```python
from build123d import *

# Parameters (mm, degrees)
SKETCH1_W           = 40
SKETCH1_H           = 20
BOSS_EXTRUDE1_DEPTH = 39
BOSS_EXTRUDE2_DEPTH = 2.5
FILLET1_R           = 2.5
SKETCH3_R           = 5
BOSS_EXTRUDE3_DEPTH = 2.5
SKETCH4_R           = 2.5
BOSS_EXTRUDE4_DEPTH = 4
FILLET2_R           = 2.5
FILLET3_R           = 2.5


with BuildPart() as part:
    # Sketch1 → Boss-Extrude1 (new body)
    with BuildSketch(Plane(origin=(0, 0, 0), x_dir=(1, 0, 0), z_dir=(0, 1, 0))):
        with Locations((20, 10)):
            Rectangle(SKETCH1_W, SKETCH1_H)
    extrude(amount=BOSS_EXTRUDE1_DEPTH)

    # Sketch2 → Boss-Extrude2 (add)
    with BuildSketch(Plane(origin=(0, 28.9, 0), x_dir=(-1, 0, 0), z_dir=(0, -1, 0))):
        with BuildLine():
            ThreePointArc((-44.8, 12.5), (-46.382129215, 13.064317395), (-47.25, 14.502506281))
            Line((-47.25, 14.502506281), (-47.25, 5.497493719))
            ThreePointArc((-47.25, 5.497493719), (-46.382129215, 6.935682605), (-44.8, 7.5))
            Line((-44.8, 7.5), (-44.8, 12.5))
        make_face()
        with BuildLine():
            Line((7.25, 20), (-47.25, 20))
            Line((-47.25, 20), (-47.25, 15.497493719))
            ThreePointArc((-47.25, 15.497493719), (-44.55, 17.487468593), (-42.3, 15))
            ThreePointArc((-42.3, 15), (-43.032233047, 13.232233047), (-44.8, 12.5))
            Line((-44.8, 12.5), (-44.8, 7.5))
            ThreePointArc((-44.8, 7.5), (-43.032233047, 6.767766953), (-42.3, 5))
            ThreePointArc((-42.3, 5), (-44.55, 2.512531407), (-47.25, 4.502506281))
            Line((-47.25, 4.502506281), (-47.25, 0))
            Line((-47.25, 0), (7.25, 0))
            Line((7.25, 0), (7.25, 4.502506281))
            ThreePointArc((7.25, 4.502506281), (2.3, 5), (7.25, 5.497493719))
            Line((7.25, 5.497493719), (7.25, 14.502506281))
            ThreePointArc((7.25, 14.502506281), (2.3, 15), (7.25, 15.497493719))
            Line((7.25, 15.497493719), (7.25, 20))
        make_face()
    extrude(amount=-BOSS_EXTRUDE2_DEPTH)

    # Fillet1
    fillet1_edges = [part.edges().sort_by_distance(p)[0] for p in [
        (47.25, 30.15, -20),
        (-7.25, 30.15, 0),
        (-7.25, 30.15, -20),
        (47.25, 30.15, 0),
    ]]
    fillet(fillet1_edges, radius=FILLET1_R)

    # Sketch3 → Boss-Extrude3 (add)
    with BuildSketch(Plane(origin=(0, 39, 0), x_dir=(1, 0, 0), z_dir=(0, 1, 0))):
        with Locations(Location((29.9, 10, 0), (0, 0, 90))):
            Circle(SKETCH3_R)
    extrude(amount=BOSS_EXTRUDE3_DEPTH)

    # Sketch4 → Boss-Extrude4 (add)
    with BuildSketch(Plane(origin=(0, 41.5, 0), x_dir=(1, 0, 0), z_dir=(0, 1, 0))):
        with Locations(Location((29.9, 10, 0), (0, 0, 270))):
            Circle(SKETCH4_R)
    extrude(amount=BOSS_EXTRUDE4_DEPTH)

    # Fillet2
    fillet2_edges = [part.edges().sort_by_distance(p)[0] for p in [
        (0, 14.45, -20),
        (40, 14.45, -20),
        (40, 14.45, 0),
        (20, 39, -20),
        (0, 14.45, 0),
        (0, 35.2, -20),
        (40, 35.2, -20),
        (40, 35.2, 0),
        (0, 35.2, 0),
        (20, 39, 0),
    ]]
    fillet(fillet2_edges, radius=FILLET2_R)

    # Fillet3
    # the kernel refuses this fillet: 2.5 mm, written as the material it takes off along each edge
    with BuildSketch(Plane(origin=(2.5, 36.5, -2.5), x_dir=(0, 1, 0), z_dir=(-1, 0, 0))) as fillet3_piece_1_section:
        Polygon((0, 0), (FILLET3_R, 0), (FILLET3_R, -FILLET3_R), (0, -FILLET3_R), align=None)
    fillet3_piece_1 = extrude(amount=FILLET3_R, mode=Mode.PRIVATE)
    fillet3_piece_1 = fillet3_piece_1 - Plane(origin=(2.5, 36.5, -2.5), x_dir=(0, -0.7071067811865475, -0.7071067811865475), z_dir=(-1, 0, 0)) * Sphere(FILLET3_R, mode=Mode.PRIVATE)
    add(fillet3_piece_1, mode=Mode.SUBTRACT)
    with BuildSketch(Plane(origin=(37.5, 36.5, -2.5), x_dir=(1, 0, 0), z_dir=(0, 1, 0))) as fillet3_piece_2_section:
        Polygon((0, 0), (FILLET3_R, 0), (FILLET3_R, -FILLET3_R), (0, -FILLET3_R), align=None)
    fillet3_piece_2 = extrude(amount=FILLET3_R, mode=Mode.PRIVATE)
    fillet3_piece_2 = fillet3_piece_2 - Plane(origin=(37.5, 36.5, -2.5), x_dir=(-0.7071067811865475, 0, -0.7071067811865475), z_dir=(0, 1, 0)) * Sphere(FILLET3_R, mode=Mode.PRIVATE)
    add(fillet3_piece_2, mode=Mode.SUBTRACT)
    with BuildSketch(Plane(origin=(37.5, 36.5, -17.5), x_dir=(1, 0, 0), z_dir=(0, 1, 0))) as fillet3_piece_3_section:
        Polygon((0, 0), (FILLET3_R, 0), (FILLET3_R, FILLET3_R), (0, FILLET3_R), align=None)
    fillet3_piece_3 = extrude(amount=FILLET3_R, mode=Mode.PRIVATE)
    fillet3_piece_3 = fillet3_piece_3 - Plane(origin=(37.5, 36.5, -17.5), x_dir=(-0.7071067811865475, 0, 0.7071067811865475), z_dir=(0, 1, 0)) * Sphere(FILLET3_R, mode=Mode.PRIVATE)
    add(fillet3_piece_3, mode=Mode.SUBTRACT)
    with BuildSketch(Plane(origin=(2.5, 36.5, -17.5), x_dir=(0, 1, 0), z_dir=(-1, 0, 0))) as fillet3_piece_4_section:
        Polygon((0, 0), (FILLET3_R, 0), (FILLET3_R, FILLET3_R), (0, FILLET3_R), align=None)
    fillet3_piece_4 = extrude(amount=FILLET3_R, mode=Mode.PRIVATE)
    fillet3_piece_4 = fillet3_piece_4 - Plane(origin=(2.5, 36.5, -17.5), x_dir=(0, -0.7071067811865475, 0.7071067811865475), z_dir=(-1, 0, 0)) * Sphere(FILLET3_R, mode=Mode.PRIVATE)
    add(fillet3_piece_4, mode=Mode.SUBTRACT)
    with BuildSketch(Plane(origin=(0, 39, -17.5), x_dir=(0, -1, 0), z_dir=(0, 0, 1))) as fillet3_piece_5:
        with BuildLine():
            CenterArc((FILLET3_R, FILLET3_R), FILLET3_R, 180, 90)
            Line((0, FILLET3_R), (0, 0))
            Line((0, 0), (FILLET3_R, 0))
        make_face()
    extrude(amount=15, mode=Mode.SUBTRACT)
    with BuildSketch(Plane(origin=(40, 39, -2.5), x_dir=(-1, 0, 0), z_dir=(0, 0, -1))) as fillet3_piece_6:
        with BuildLine():
            CenterArc((FILLET3_R, -FILLET3_R), FILLET3_R, 90, 90)
            Line((0, -FILLET3_R), (0, 0))
            Line((0, 0), (FILLET3_R, 0))
        make_face()
    extrude(amount=15, mode=Mode.SUBTRACT)


solid = part.part
```
Can you work these out from the model? Positions are in its coordinate system, mm. A direction names the side the tool comes from. Give positions to 0.01 mm unless a question says otherwise; leave off trailing zeros. Loops run counter-clockwise (first coordinate to the right, second up) from the corner with the lowest first, then second, coordinate; pieces in that order, holes last. Notation, with made-up numbers: M 87,12.25 L 134,12.25 A8 cw 134,16.25 Z; hole C 15.5,20.5 d1. An arc over 180 degrees is marked long. Use one line per item in the form item = value. Start each with the question number.
(1) I want a section at C-C, the plane x = 29.9. Write out the boundary of the cut face in (y, z), and give its area (3 significant figures).
(2) On a 3-axis mill with a long thin cutter (end or side, diameter ignored), from which of +Z, -Z, +X, -X, +Y, -Y can I reach the whole of each face in a straight line? I mean faces 1 (the cylindrical face through (32.38, 43.47, -10.33)), 2 (the cylindrical face through (0.752, 14.652, -0.713)), 3 (the cylindrical face through (39.248, 33.986, -0.713)). Say none if no direction works.
(3) I'm going to push flat-ended pins straight in: P1, Ø4.5, axis at y = 10, z = -12.5, coming from the +X side; P2, Ø12, axis at x = 14, z = -6.5, coming from the +Y side; P3, Ø1, axis at x = -1.5, z = -11, coming from the -Y side; P4, Ø4, axis at x = -4.8, z = -15, coming from the -Y side. Where does each tip first touch, or does it pass through?
(4) Please list where these lines run through material, in increasing order: line 1 (Z direction, x = -4.8, y = 30); line 2 (Z direction, x = -4, y = 29); line 3 (X direction, y = 30.6, z = -15).
(5) I want a section at D-D, the plane z = -10. Write out the boundary of the cut face in (x, y).
(6) I want a section at B-B, the plane z = -6.25. Write out the boundary of the cut face in (x, y), and give its area (3 significant figures).
(7) I want a section at A-A, the plane y = 30.5. Write out the boundary of the cut face in (x, z).
(8) Thinking about a two-plate mould opening in Y: for faces 4 (the cylindrical face through (20.245, 38.248, -0.713)), 5 (the flat face through (20, 18, -20)), which applies, released by +Y, released by -Y, zero draft, split by the parting line, or undercut?
Worked out:
q1.outline = M 0,-20 L 36.5,-20 A2.5 ccw 39,-17.5 L 39,-15 L 41.5,-15 L 41.5,-12.5 L 45.5,-12.5 L 45.5,-7.5 L 41.5,-7.5 L 41.5,-5 L 39,-5 L 39,-2.5 A2.5 ccw 36.5,0 L 0,0 Z
q1.area = 822 mm²
q2.face_1 = +Y
q2.face_2 = +Z, -X, -Y
q2.face_3 = +Z, +X, +Y
q3.P1 = 40
q3.P2 = 39
q3.P3 = 28.9
q3.P4 = through
q4.line_1 = -20 to -17.5, -12.5 to -7.5, -2.5 to 0
q4.line_2 = -20 to -17.37, -12.63 to -7.37, -2.63 to 0
q4.line_3 = -2.3 to 42.3
q5.outline = M -7.25,28.9 L 0,28.9 L 0,0 L 40,0 L 40,28.9 L 47.25,28.9 L 47.25,31.4 L 40,31.4 L 40,36.5 A2.5 ccw 37.5,39 L 34.9,39 L 34.9,41.5 L 32.4,41.5 L 32.4,45.5 L 27.4,45.5 L 27.4,41.5 L 24.9,41.5 L 24.9,39 L 2.5,39 A2.5 ccw 0,36.5 L 0,31.4 L -7.25,31.4 Z
q6.outline = M -7.25,28.9 L -6.97,28.9 L -6.97,31.4 L -7.25,31.4 Z; M -2.63,28.9 L 0,28.9 L 0,0 L 40,0 L 40,28.9 L 42.63,28.9 L 42.63,31.4 L 40,31.4 L 40,36.5 A2.5 ccw 37.5,39 L 33.21,39 L 33.21,41.5 L 26.59,41.5 L 26.59,39 L 2.5,39 A2.5 ccw 0,36.5 L 0,31.4 L -2.63,31.4 Z; M 46.97,28.9 L 47.25,28.9 L 47.25,31.4 L 46.97,31.4 Z
q6.area = 1,590 mm²
q7.outline = M -7.25,-17.5 A2.5 ccw -4.75,-20 L 44.75,-20 A2.5 ccw 47.25,-17.5 L 47.25,-15.5 A2.5 cw long 47.25,-14.5 L 47.25,-5.5 A2.5 cw long 47.25,-4.5 L 47.25,-2.5 A2.5 ccw 44.75,0 L -4.75,0 A2.5 ccw -7.25,-2.5 L -7.25,-4.5 A2.5 cw long -7.25,-5.5 L -7.25,-14.5 A2.5 cw long -7.25,-15.5 Z
q8.face_4 = released by +Y
q8.face_5 = zero draft
